Verification items for the finished model (mm, model axes). Face numbers are marked on the shaded views. A direction names the side the tool comes from. Round coordinates to 2 decimals unless told otherwise and drop trailing zeros. Order: outer loops, then holes, each group sorted by start corner. A loop starts at its lowest first (then second) coordinate and runs counter-clockwise, first axis right, second up. Notation, with made-up numbers: (-20.75, -28) -> (6.25, -28) arc R15 cw to (6.25, -7) -> close; hole circle Ø10 at (49.25, -29). An arc over 180 degrees is marked (long way). Answer in a Markdown table with one row per item. Add a question column.
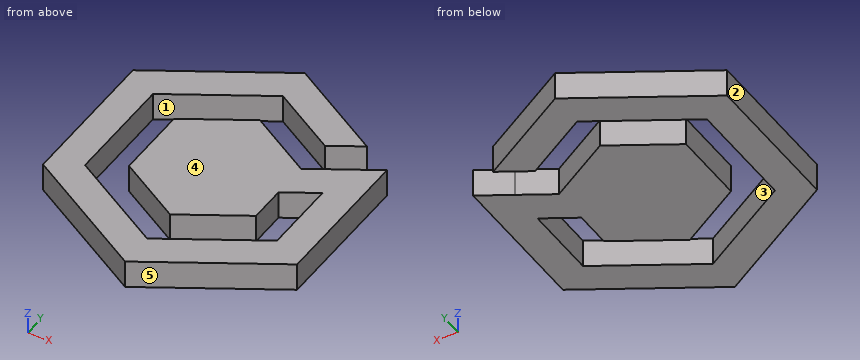
```python
from build123d import *

# Parameters (mm, degrees)
F1_DEPTH = 5


with BuildPart() as f1:
    # F0 (on Top) → F1 (new body)
    with BuildSketch(Plane.XY):
        Polygon((-22.5, -12.990381), (0, -25.980762), (0, -19.629909), (-17, -9.814955), (-17, 9.814955), (-22.5, 12.990381), align=None)
        Polygon((11.5, 12.990381), (17, 16.165808), (0, 25.980762), (-22.5, 12.990381), (-17, 9.814955), (0, 19.629909), align=None)
        Polygon((22.5, -12.990381), (22.5, 12.990381), (17, 9.814955), (17, 3.319764), (17, -9.814955), (0, -19.629909), (0, -25.980762), align=None)
        Polygon((0, 0), (11.25, 6.495191), (0, 12.990381), (-11.25, 6.495191), align=None)
        Polygon((0, -12.990381), (0, 0), (-11.25, 6.495191), (-11.25, -6.495191), align=None)
        Polygon((11.25, 0), (11.25, 6.495191), (0, 0), (0, -12.990381), (11.25, -6.495191), align=None)
        Polygon((17, 3.319764), (17, 9.814955), (11.25, 6.495191), (11.25, 0), align=None)
    extrude(amount=F1_DEPTH)


solid = f1.part
```
1) Cross-section at C-C, the plane x = 1.5. Record the boundary of the cut face in (y, z), and give its area (3 significant figures).
2) Cross-section at D-D, the plane x = -16. Record the boundary of the cut face in (y, z), and give its area (3 significant figures).
3) Cross-section at B-B, the plane z = 1.25. Record the boundary of the cut face in (x, y), and give its area (3 significant figures).
4) Draft check along X on the marked faces 3, 4 and 5. Enter one of: +X half, -X half, draft (parallel to the pull), parting line (faces both ways), or undercut.
5) Thickness scan on L1, parallel to X at y = -5.5, z = 2.5; L2, parallel to Y at x = -4, z = 1.1; L3, parallel to Y at x = 8, z = 4.55. Record the ranges inside material, lowest first. Write a range as [from, to].
6) Tool access check on the marked faces 1 and 2. Record the directions out of +Z, -Z, +X, -X, +Y, -Y that give a thin tool (end or side, any length) a straight path to the whole face; none if there is none.
7) Cross-section at A-A, the plane y = -3. Record the boundary of the cut face in (x, z).
Results below:
| question | item | result |
|---|---|---|
| 1 | outline | (-25.11, 0) -> (-18.76, 0) -> (-18.76, 5) -> (-25.11, 5) -> close; (-12.12, 0) -> (12.12, 0) -> (12.12, 5) -> (-12.12, 5) -> close; (18.76, 0) -> (25.11, 0) -> (25.11, 5) -> (18.76, 5) -> close |
| 1 | area | 185 mm² |
| 2 | outline | (-16.74, 0) -> (-10.39, 0) -> (-10.39, 5) -> (-16.74, 5) -> close; (10.39, 0) -> (16.74, 0) -> (16.74, 5) -> (10.39, 5) -> close |
| 2 | area | 63.5 mm² |
| 3 | outline | (-22.5, -12.99) -> (0, -25.98) -> (22.5, -12.99) -> (22.5, 12.99) -> (11.25, 6.5) -> (0, 12.99) -> (-11.25, 6.5) -> (-11.25, -6.5) -> (0, -12.99) -> (11.25, -6.5) -> (11.25, 0) -> (17, 3.32) -> (17, -9.81) -> (0, -19.63) -> (-17, -9.81) -> (-17, 9.81) -> (0, 19.63) -> (11.5, 12.99) -> (17, 16.17) -> (0, 25.98) -> (-22.5, 12.99) -> close |
| 3 | area | 1,190 mm² |
| 4 | face 3 | undercut |
| 4 | face 4 | draft |
| 4 | face 5 | +X half |
| 5 | L1 | [-22.5, -17], [-11.25, 11.25], [17, 22.5] |
| 5 | L2 | [-23.67, -17.32], [-10.68, 10.68], [17.32, 23.67] |
| 5 | L3 | [-21.36, -15.01], [-8.37, 8.37], [15.01, 21.36] |
| 6 | face 1 | +Z, -Z |
| 6 | face 2 | +Z, -Z, -X, +Y, -Y |
| 7 | outline | (-22.5, 0) -> (-17, 0) -> (-17, 5) -> (-22.5, 5) -> close; (-11.25, 0) -> (11.25, 0) -> (11.25, 5) -> (-11.25, 5) -> close; (17, 0) -> (22.5, 0) -> (22.5, 5) -> (17, 5) -> close |
